Could you check a few things on this model? Use its own coordinates, in mm. Round coordinates to 2 decimals unless told otherwise and drop trailing zeros. Write each loop counter-clockwise with the first axis right and the second up, starting at its lowest first coordinate (ties: lowest second). Pieces come first, ordered by that corner, then holes. Notation, with made-up numbers: (26.25, -11) -> (61.25, -11) arc R30 cw to (61.25, 23) -> close; hole circle Ø11 at (-16, -7.75). An arc over 180 degrees is marked (long way). Return JSON: item names as keys, results as strings.
from build123d import *

# Parameters (mm, degrees)
BOSS_EXTRUDE2_DEPTH = 0.5
SKETCH3_R           = 0.65
CUT_EXTRUDE3_DEPTH  = 0.5


with BuildPart() as part:
    # Sketch1 → Boss-Extrude2 (new body)
    with BuildSketch(Plane(origin=(0, 0, 0), x_dir=(1, 0, 0), z_dir=(0, 1, 0))):
        Polygon((-1, 7), (1, 7), (1.4, 6.6), (1.4, -0.065616498), (0.65, 0), (0.55, -2.95), (0, -3.5), (-0.55, -2.95), (-0.65, 0), (-1.4, -0.065616498), (-1.4, 6.6), align=None)
    extrude(amount=BOSS_EXTRUDE2_DEPTH)

    # Sketch3 → Cut-Extrude3 (cut)
    with BuildSketch(Plane(origin=(0, 0.5, 0), x_dir=(1, 0, 0), z_dir=(0, 1, 0))):
        with Locations(Location((0, 4.8, 0), (0, 0, 270))):
            Circle(SKETCH3_R)
    extrude(amount=-CUT_EXTRUDE3_DEPTH, mode=Mode.SUBTRACT)


solid = part.part
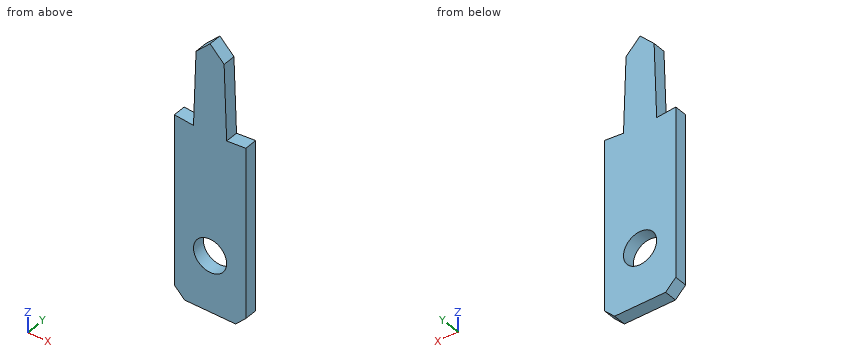
1) I want a section at D-D, the plane z = 1.25. Please give me the cut outline in (x, y).
Return value:
{"outline": "(-0.61, 0) -> (0.61, 0) -> (0.61, 0.5) -> (-0.61, 0.5) -> close"}
2) I want a section at A-A, the plane z = -4.8. Please give me the cut outline in (x, y).
Return value:
{"outline": "(-1.4, 0) -> (-0.65, 0) -> (-0.65, 0.5) -> (-1.4, 0.5) -> close; (0.65, 0) -> (1.4, 0) -> (1.4, 0.5) -> (0.65, 0.5) -> close"}
3) I want a section at B-B, the plane x = 0.35. Please give me the cut outline in (y, z), and give its area (3 significant figures).
Return value:
{"outline": "(0, -7) -> (0.5, -7) -> (0.5, -5.35) -> (0, -5.35) -> close; (0, -4.25) -> (0.5, -4.25) -> (0.5, 3.15) -> (0, 3.15) -> close", "area": "4.53 mm²"}
4) I want a section at C-C, the plane y = 0.3. Please give me the cut outline in (x, z).
Return value:
{"outline": "(-1.4, -6.6) -> (-1, -7) -> (1, -7) -> (1.4, -6.6) -> (1.4, 0.07) -> (0.65, 0) -> (0.55, 2.95) -> (0, 3.5) -> (-0.55, 2.95) -> (-0.65, 0) -> (-1.4, 0.07) -> close; hole circle Ø1.3 at (0, -4.8)"}
5) If I drill on probe 1 along X at (y, z) = (0.1, -4.8); probe 2 along Z at (x, y) = (0.25, 0.1); probe 3 along X at (y, z) = (0.1, -4.25), over which ranges is the centre line in solid material (lowest first)? Write a range as [from, to].
Return value:
{"probe 1": "[-1.4, -0.65], [0.65, 1.4]", "probe 2": "[-7, -5.4], [-4.2, 3.25]", "probe 3": "[-1.4, -0.35], [0.35, 1.4]"}
